Read the model definition and answer for the solid it produces. Units are mm, in the model's axes. A direction names the side the tool comes from. Round coordinates to 2 decimals unless told otherwise and drop trailing zeros. Order: outer loops, then holes, each group sorted by start corner. A loop starts at its lowest first (then second) coordinate and runs counter-clockwise, first axis right, second up. Notation, with made-up numbers: (-30, 21.5) - (23, 21.5) arc R25 cw to (23, 57.5) - close; hole circle Ø1 at (48, -14). An arc over 180 degrees is marked (long way). Put each result on its own line as item: value. Start each with the question number.
Q1. Section B-B on y = 6 is taken. Give the vertices of the cut face in (x, z).
Q2. Which of the six approach directions +Z, -Z, +X, -X, +Y, -Y give full straight-line access (tool end or side, diameter ignored) to faces 5 (the face through (-7.65, 0.07, 2.46)), 6 (the face through (17, 3, 2))?
Q3. Find the intervals of material crossed by line 1 along Y through (x, z) = (0, 2.65); line 2 along X through (y, z) = (4.75, 4.7); line 3 along Y through (x, z) = (6, 1.35), in increasing order. Write a range as from..to.
Q4. Section A-A on x = 0 is taken. Give the vertices of the cut face in (y, z), then the cut area to 3 significant figures.
Q5. For a pull along X with two mould halves and no side action, classify faces 1 (the face through (26.567, -2.465, 2.465)), 2 (the face through (5, -2, 0)), 3 (the face through (24.539, -4, 2)), 4 (the face through (17, -3, 2)) as pulls with the +X half, pulls with the -X half, needs draft (parallel to the pull), parting line crosses it, or undercut.
Q6. Each of these flat-tipped pins is pushed along its axis until it touches: pin 1 Ø1 at (y, z) = (5.5, 3) entering from -X; pin 2 Ø0.6 at (y, z) = (-3.5, 2.5) entering from -X; pin 3 Ø0.6 at (y, z) = (4, 2) entering from -X. Where does it stop, or does it pass through?
Q7. Section C-C on z = 2.25 is taken. Give the vertices of the cut face in (x, y), then the cut area to 3 significant figures.
from build123d import *

# Parameters (mm, degrees)
SKETCH1_R           = 2
SKETCH1_R_2         = 1.65
BOSS_EXTRUDE1_DEPTH = 5


with BuildPart() as part:
    # Sketch1 → Boss-Extrude1 (new body)
    with BuildSketch(Plane.XY):
        with BuildLine():
            Line((9.539392014, 3), (24.539392014, 3))
            Line((24.539392014, 3), (24.539392014, 5))
            Line((24.539392014, 5), (28.539392014, 0))
            Line((28.539392014, 0), (24.539392014, -5))
            Line((24.539392014, -5), (24.539392014, -3))
            Line((24.539392014, -3), (9.539392014, -3))
            ThreePointArc((9.539392014, -3), (-10, 0), (9.539392014, 3))
        make_face()
        Circle(SKETCH1_R, mode=Mode.SUBTRACT)
        with Locations((0, 6)):
            Circle(SKETCH1_R_2, mode=Mode.SUBTRACT)
        with Locations((6, 0)):
            Circle(SKETCH1_R_2, mode=Mode.SUBTRACT)
        with Locations((0, -6)):
            Circle(SKETCH1_R_2, mode=Mode.SUBTRACT)
        with Locations((-6, 0)):
            Circle(SKETCH1_R_2, mode=Mode.SUBTRACT)
    extrude(amount=BOSS_EXTRUDE1_DEPTH)


solid = part.part
Findings:
1. outline: (-8, 0) - (-1.65, 0) - (-1.65, 5) - (-8, 5) - close; (1.65, 0) - (8, 0) - (8, 5) - (1.65, 5) - close
2. face 5: +Z, -Z
2. face 6: +Z, -Z, +Y
3. line 1: -10..-7.65, -4.35..-2, 2..4.35, 7.65..10
3. line 2: -8.8..-1.08, 1.08..8.8, 24.54..24.74
3. line 3: -8..-1.65, 1.65..8
4. outline: (-10, 0) - (-7.65, 0) - (-7.65, 5) - (-10, 5) - close; (-4.35, 0) - (-2, 0) - (-2, 5) - (-4.35, 5) - close; (2, 0) - (4.35, 0) - (4.35, 5) - (2, 5) - close; (7.65, 0) - (10, 0) - (10, 5) - (7.65, 5) - close
4. area: 47.0 mm2
5. face 1: pulls with the +X half
5. face 2: needs draft
5. face 3: undercut
5. face 4: undercut
6. pin 1: x = -8.66
6. pin 2: x = -9.47
6. pin 3: x = -9.29
7. outline: (9.54, -3) - (24.54, -3) - (24.54, -5) - (28.54, 0) - (24.54, 5) - (24.54, 3) - (9.54, 3) arc R10 ccw (long way) to start; hole circle Ø3.3 at (-6, 0); hole circle Ø4 at (0, 0); hole circle Ø3.3 at (0, -6); hole circle Ø3.3 at (0, 6); hole circle Ø3.3 at (6, 0)
7. area: 376 mm2
